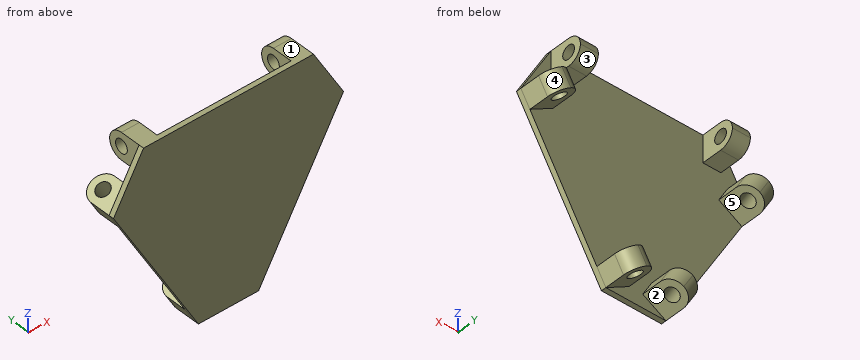
```python
from build123d import *

# Parameters (mm, degrees)
BOSS_EXTRUDE2_DEPTH      = 1.5
SKETCH4_W                = 5.364695745
SKETCH4_H                = 8
BOSS_EXTRUDE3_DEPTH      = 10
SKETCH5_R                = 2
CUT_EXTRUDE2_DEPTH       = 70.885624116
FILLET1_R                = 4
CIRPATTERN1_COUNT        = 3
FILLET1_OF_CIRPATTERN1_R = 4


with BuildPart() as part:
    # Sketch3 → Boss-Extrude2 (new body)
    with BuildSketch(Plane(origin=(0, 0, 0), x_dir=(1, 0, 0), z_dir=(0, 1, 0))):
        Polygon((-8.968287222, 34.466470874), (8.968287222, 34.466470874), (34.332982967, -9.466470874), (25.364695745, -25), (-25.364695745, -25), (-34.332982967, -9.466470874), align=None)
    extrude(amount=BOSS_EXTRUDE2_DEPTH)

    # Sketch4 → Boss-Extrude3 (add)
    with BuildSketch(Plane(origin=(0, 1.5, 0), x_dir=(1, 0, 0), z_dir=(0, 1, 0))):
        with Locations((-22.682347873, -21)):
            Rectangle(SKETCH4_W, SKETCH4_H)
        with Locations((22.682347873, -21)):
            Rectangle(SKETCH4_W, SKETCH4_H)
    boss_extrude3 = extrude(amount=BOSS_EXTRUDE3_DEPTH)

    # Sketch5 → Cut-Extrude2 (cut, through all)
    with BuildSketch(Plane(origin=(25.364695745, 0, 0), x_dir=(0, 0, -1), z_dir=(1, 0, 0))):
        with Locations((-21, 7.5)):
            Circle(SKETCH5_R)
    cut_extrude2 = extrude(amount=-CUT_EXTRUDE2_DEPTH, mode=Mode.SUBTRACT)

    # Fillet1
    fillet1_edges = [part.edges().sort_by_distance(p)[0] for p in [
        (-22.682347872, 11.5, 17),
        (-22.682347872, 11.5, 25),
        (22.682347872, 11.5, 17),
        (22.682347872, 11.5, 25),
    ]]
    fillet(fillet1_edges, radius=FILLET1_R - 0.0001)  # a hair under: the kernel refuses the full size

    # CirPattern1: Boss-Extrude3, Cut-Extrude2 ×3 about axis
    cirpattern1_axis = Axis((0, 0, 0), (0, 1, 0))
    add([boss_extrude3.rotate(cirpattern1_axis, i * 360 / CIRPATTERN1_COUNT) for i in range(1, CIRPATTERN1_COUNT)])
    add([cut_extrude2.rotate(cirpattern1_axis, i * 360 / CIRPATTERN1_COUNT) for i in range(1, CIRPATTERN1_COUNT)], mode=Mode.SUBTRACT)

    # Fillet1 of CirPattern1
    fillet1_of_cirpattern1_edges = [part.edges().sort_by_distance(p)[0] for p in [
        (26.063605801, 11.5, 11.143489475),
        (32.991809031, 11.5, 7.143489475),
        (3.381257928, 11.5, -28.143489475),
        (10.309461158, 11.5, -32.143489475),
        (-3.381257928, 11.5, -28.143489475),
        (-10.309461158, 11.5, -32.143489475),
        (-26.063605801, 11.5, 11.143489475),
        (-32.991809031, 11.5, 7.143489475),
    ]]
    fillet(fillet1_of_cirpattern1_edges, radius=FILLET1_OF_CIRPATTERN1_R - 0.0001)  # a hair under: the kernel refuses the full size


solid = part.part
```
Source: CAD feature listing. Evaluate the final solid. Frame: model axes, mm. Face numbers are marked on the shaded views. A direction names the side the tool comes from. Coordinates: 2 decimals unless noted, no trailing zeros. Loops run counter-clockwise (first coordinate to the right, second up) from the corner with the lowest first, then second, coordinate; pieces in that order, holes last. Notation, with made-up numbers: M 46,53 L 70,53 A16 cw 70,71 Z; hole C -22.5,-38.75 d10. An arc over 180 degrees is marked long. Use a Markdown table: item, result. Add a question column.
Q1. Access query for the marked faces 1 and 2. Directions: +Z, -Z, +X, -X, +Y, -Y. A direction counts if a zero-diameter tool reaches every point of the face in a straight line with its end or side. Return the directions, or none.
Q2. Section query C-C, the plane z = -19. Return loops of the section in (x, y), and give its area (3 significant figures).
Q3. Section query A-A, the plane y = 3.25. Return loops of the section in (x, z).
Q4. First-contact query: pin 1 (4 mm diameter, centred on y = 2.5, z = -3, fed in from -X); pin 2 (3.5 mm diameter, centred on y = 7.5, z = 21, fed in from +X); pin 3 (1.6 mm diameter, centred on x = -22.5, y = 4.5, fed in from -Z); pin 4 (4 mm diameter, centred on y = 7.5, z = 20, fed in from -X). Flat tips, straight axial feed; report the tip coordinate or a pass-through.
Q5. Draft query along X for the marked faces 3, 4 and 5. Return one class per face: pulls with the +X half, pulls with the -X half, needs draft (parallel to the pull), parting line crosses it, or undercut.
Q6. Material intervals for L1, parallel to Z at x = -20.5, y = 7.25; L2, parallel to Y at x = -22, z = 21; L3, parallel to X at y = 5.75, z = 9, sorted ascending.
Result:
| question | item | result |
|---|---|---|
| 1 | face 1 | +Z, +X, -X, +Y, -Y |
| 1 | face 2 | -Z, +Y |
| 2 | outline | M -17.9,0 L 17.9,0 L 17.9,1.5 L -17.9,1.5 Z |
| 2 | area | 53.7 mm2 |
| 3 | outline | M -34.33,9.47 L -31.65,4.82 L -24.72,8.82 L -27.4,13.47 Z; M -25.36,17 L -20,17 L -20,25 L -25.36,25 Z; M -11.65,-29.82 L -8.97,-34.47 L -2.04,-30.47 L -4.72,-25.82 Z; M 2.04,-30.47 L 8.97,-34.47 L 11.65,-29.82 L 4.72,-25.82 Z; M 20,17 L 25.36,17 L 25.36,25 L 20,25 Z; M 24.72,8.82 L 31.65,4.82 L 34.33,9.47 L 27.4,13.47 Z |
| 4 | pin 1 | stops at x = -28.14 |
| 4 | pin 2 | passes through |
| 4 | pin 3 | stops at z = 17 |
| 4 | pin 4 | stops at x = -25.36 |
| 5 | face 3 | needs draft |
| 5 | face 4 | pulls with the +X half |
| 5 | face 5 | undercut |
| 6 | L1 | z = 17 to 19.02, 22.98 to 25 |
| 6 | L2 | y = 0 to 5.5, 9.5 to 11.5 |
| 6 | L3 | x = -34.06 to -30.56, -28.33 to -24.83, 24.83 to 28.33, 30.56 to 34.06 |
